```python
from build123d import *

# Parameters (mm, degrees)
CROQUIS1_R              = 1.55
CROQUIS1_R_2            = 2.55
CROQUIS1_R_3            = 2.5
CROQUIS1_W              = 3.2
CROQUIS1_H              = 6
SALIENTE_EXTRUIR1_DEPTH = 3
REDONDEO2_R             = 2


with BuildPart() as part:
    # Croquis1 → Saliente-Extruir1 (new body)
    with BuildSketch(Plane(origin=(0, 0, 0), x_dir=(1, 0, 0), z_dir=(0, 1, 0))):
        Polygon((0, 0), (375, 0), (375, 31), (329.4, 31), (329.4, 39), (315.4, 39), (315.4, 31), (59.6, 31), (59.6, 39), (45.6, 39), (45.6, 31), (0, 31), align=None)
        with Locations((5, 15)):
            Circle(CROQUIS1_R, mode=Mode.SUBTRACT)
        with Locations((370, 15)):
            Circle(CROQUIS1_R, mode=Mode.SUBTRACT)
        with Locations((10, 27.1)):
            Circle(CROQUIS1_R_2, mode=Mode.SUBTRACT)
        with Locations((33.2, 27.1)):
            Circle(CROQUIS1_R_2, mode=Mode.SUBTRACT)
        with Locations((33.2, 3.9)):
            Circle(CROQUIS1_R_2, mode=Mode.SUBTRACT)
        with Locations((10, 3.9)):
            Circle(CROQUIS1_R_2, mode=Mode.SUBTRACT)
        with Locations((365, 3.9)):
            Circle(CROQUIS1_R_2, mode=Mode.SUBTRACT)
        with Locations((341.8, 3.9)):
            Circle(CROQUIS1_R_2, mode=Mode.SUBTRACT)
        with Locations((365, 27.1)):
            Circle(CROQUIS1_R_2, mode=Mode.SUBTRACT)
        with Locations((341.8, 27.1)):
            Circle(CROQUIS1_R_2, mode=Mode.SUBTRACT)
        with Locations((189, 25)):
            Circle(CROQUIS1_R, mode=Mode.SUBTRACT)
        with Locations((189, 5)):
            Circle(CROQUIS1_R, mode=Mode.SUBTRACT)
        with Locations((52.6, 22)):
            Circle(CROQUIS1_R, mode=Mode.SUBTRACT)
        with Locations((52.6, 4)):
            Circle(CROQUIS1_R, mode=Mode.SUBTRACT)
        with Locations((322.4, 22)):
            Circle(CROQUIS1_R, mode=Mode.SUBTRACT)
        with Locations((322.4, 4)):
            Circle(CROQUIS1_R, mode=Mode.SUBTRACT)
        with Locations((312.4, 26)):
            Circle(CROQUIS1_R, mode=Mode.SUBTRACT)
        with Locations((301.4, 26)):
            Circle(CROQUIS1_R, mode=Mode.SUBTRACT)
        with Locations((306.9, 18)):
            Circle(CROQUIS1_R_3, mode=Mode.SUBTRACT)
        with Locations((370, 4.5)):
            Rectangle(CROQUIS1_W, CROQUIS1_H, mode=Mode.SUBTRACT)
        with Locations((5, 25.5)):
            Rectangle(CROQUIS1_W, CROQUIS1_H, mode=Mode.SUBTRACT)
        with Locations((5, 4.5)):
            Rectangle(CROQUIS1_W, CROQUIS1_H, mode=Mode.SUBTRACT)
        with Locations((370, 25.5)):
            Rectangle(CROQUIS1_W, CROQUIS1_H, mode=Mode.SUBTRACT)
    extrude(amount=SALIENTE_EXTRUIR1_DEPTH)

    # Redondeo2
    redondeo2_edges = [part.edges().sort_by_distance(p)[0] for p in [
        (0, 1.5, -31),
        (45.6, 1.5, -31),
        (45.6, 1.5, -39),
        (59.6, 1.5, -39),
        (59.6, 1.5, -31),
        (315.4, 1.5, -31),
        (315.4, 1.5, -39),
        (329.4, 1.5, -39),
        (329.4, 1.5, -31),
        (375, 1.5, -31),
        (375, 1.5, 0),
        (0, 1.5, 0),
    ]]
    fillet(redondeo2_edges, radius=REDONDEO2_R)


solid = part.part
```
Model file for the job. Use its own axes, mm. Coordinates: 2 decimals unless noted, no trailing zeros. Loops run counter-clockwise (first coordinate to the right, second up) from the corner with the lowest first, then second, coordinate; pieces in that order, holes last. Notation, with made-up numbers: (15.5, -36) - (64.5, -36) arc R12 cw to (64.5, -25) - close; hole circle Ø7 at (-15, -20.5). An arc over 180 degrees is marked (long way). Answer as a JSON object with one key per item and string values. Group by question number.
(1) Flat gauge pins, fed straight in: pin 1 (1 mm diameter, centred on x = 232.5, y = 1.5, fed in from -Z); pin 2 (1.9 mm diameter, centred on x = 322.4, z = -4, fed in from -Y). Where does each tip first touch, or does it go through?
(2) Probe line 1 along Z through (x, y) = (322.4, 2.1); line 2 along Z through (x, y) = (33.2, 0.6); line 3 along X through (y, z) = (1.6, -32.5). List the from-to ranges inside material, lowest first.
(3) Cut at B-B (y = 1.1). State how many separate pieces and enclosed holes the cut face has, then the cut area to 3 significant figures.
(4) Cut at A-A (x = 248.5). Give the cut face in (y, z), then the cut area to 3 significant figures.
Geometry says:
{
 "1": {"pin 1": "stops at z = -31", "pin 2": "passes through"},
 "2": {"line 1": "z = -39 to -23.55, -20.45 to -5.55, -2.45 to 0", "line 2": "z = -31 to -29.65, -24.55 to -6.45, -1.35 to 0", "line 3": "x = 45.54 to 59.66, 315.34 to 329.46"},
 "3": {"separate pieces": "1", "enclosed holes": "23", "area": "11,500 mm^2"},
 "4": {"outline": "(0, -31) - (3, -31) - (3, 0) - (0, 0) - close", "area": "93.0 mm^2"}
}
